The model under review builds one solid part; all positions refer to its coordinate system, in mm. Face numbers are marked on the shaded views. A direction names the side the tool comes from. Coordinates: 2 decimals unless noted, no trailing zeros. Loops run counter-clockwise (first coordinate to the right, second up) from the corner with the lowest first, then second, coordinate; pieces in that order, holes last. Notation, with made-up numbers: M 57.25,-20 L 82.25,-20 A28 ccw 82.25,11 Z; hole C 20.5,26 d6. An arc over 180 degrees is marked long. Use one line per item in the form item = value.
```python
from build123d import *

# Parameters (mm, degrees)
F1_DEPTH = 6.2484
F3_DEPTH = 0.9398
F4_W     = 24.0350353877
F4_H     = 1.27
F5_DEPTH = 1.27
F7_DEPTH = 9.145


with BuildPart() as f1:
    # F0 (on Top) → F1 (new body)
    with BuildSketch(Plane.XY):
        with BuildLine():
            Line((10.287, 4.572), (-23.3934, 4.572))
            Line((-23.3934, 4.572), (-23.3934, -4.572))
            Line((-23.3934, -4.572), (10.287, -4.572))
            ThreePointArc((10.287, -4.572), (14.859, 0), (10.287, 4.572))
        make_face()
    extrude(amount=F1_DEPTH)

    # F2 (on face) → F3 (cut)
    with BuildSketch(Plane(origin=(0, 4.572, 0), x_dir=(-1, 0, 0), z_dir=(0, 1, 0))):
        Polygon((23.3934, 6.2484), (-2.0066, 6.2484), (-0.6416353877, 4.064), (23.3934, 4.064), align=None)
    extrude(amount=-F3_DEPTH, mode=Mode.SUBTRACT)

    # F4 (on face) → F5 (cut)
    with BuildSketch(Plane(origin=(0, 3.6322, 0), x_dir=(-1, 0, 0), z_dir=(0, 1, 0))):
        with Locations((11.3758823062, 4.699)):
            Rectangle(F4_W, F4_H)
    extrude(amount=-F5_DEPTH, mode=Mode.SUBTRACT)

    # F6 (on face) → F7 (cut, through all)
    with BuildSketch(Plane(origin=(0, 4.572, 0), x_dir=(-1, 0, 0), z_dir=(0, 1, 0))):
        Polygon((19.4889663415, 6.2484), (23.3934, 0), (23.3934, 6.2484), align=None)
    extrude(amount=-F7_DEPTH, mode=Mode.SUBTRACT)

    # F8: F1 across plane


with BuildPart() as f1_1:
    add(f1.part)
    add(f1.part.mirror(Plane.XZ), mode=Mode.INTERSECT)

    # F9 (on Front) → F10 (revolve, cut)
    with BuildSketch(Plane.XZ):
        Polygon((3.4612531172, 5.5391628772), (0, 0), (-1.3459949312, -2.1540421642), (-0.3228249031, -2.7933897565), (4.4844231452, 4.8998152849), align=None)
        Polygon((5.7204784574, 9.154679198), (3.4612531172, 5.5391628772), (4.4844231452, 4.8998152849), (7.6917084592, 4.9278048398), (9.0377033903, 7.081847004), align=None)
    revolve(axis=Axis((2.8602392287, 0, 4.577339599), (0.5299192642, 0, 0.8480480962)), mode=Mode.SUBTRACT)


solid = f1_1.part
```
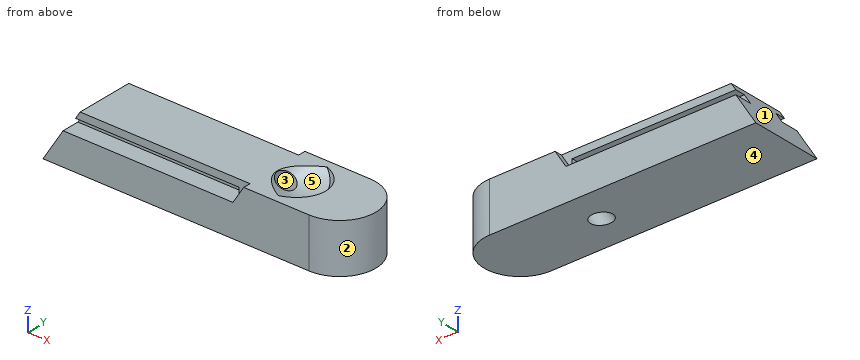
1. Add section C-C (x = 12.5). State the section outline as (y, z) points, then the cut area to 3 significant figures.
Response values:
outline = M -4,0 L 4,0 L 4,6.25 L -4,6.25 Z
area = 50.0 mm^2
2. Insertion check: P1, Ø1.4, axis at y = 3, z = 4.5, coming from the -X side; P2, Ø1.7, axis at x = -5, z = 5.5, coming from the -Y side; P3, Ø0.6, axis at x = -11, z = 4.5, coming from the -Y side. Each pin has a flat end and moves straight along its axis. Give the tip position at first contact, or say it passes through.
Response values:
P1 = -21.02
P2 = -3.63
P3 = -2.36
3. The part is to be moulded in two halves that separate along Y. For the marked faces 1, 2 and 3, say which applies: pulls with the +Y half, pulls with the -Y half, needs draft (parallel to the pull), parting line crosses it, or undercut.
Response values:
face_1 = needs draft
face_2 = parting line crosses it
face_3 = undercut
4. Add section A-A (y = 0). State the section outline as (x, z) points.
Response values:
outline = M -23.39,0 L -1.42,0 L 2.44,6.18 L 2.4,6.25 L -19.49,6.25 Z; M 1.42,0 L 14.86,0 L 14.86,6.25 L 8.52,6.25 L 7.69,4.93 L 4.48,4.9 Z
5. Wall thickness on line 1 along Z through (x, y) = (-0.5, 2.75); line 2 along X through (y, z) = (0.75, 4.5); line 3 along X through (y, z) = (0.25, 5.5): over which ranges is each line inside the solid? List them lowest first. Write a range as from..to.
Response values:
line_1 = 0..4.06, 5.33..6.25
line_2 = -20.58..1.7, 3.93..14.8
line_3 = -19.96..2.04, 8.04..14.85
6. Machinability: for the marked faces 4 and 5, which of the approach directions +Z, -Z, +X, -X, +Y, -Y give a long, thin tool a straight path to every point of the face, cutting with its end or side? Answer none if there is none.
Response values:
face_4 = -Z, +X, -X, +Y, -Y
face_5 = +Z
7. Add section B-B (x = -13). State the section outline as (y, z) points.
Response values:
outline = M -4.57,0 L 4.57,0 L 4.57,4.06 L 2.36,4.06 L 2.36,5.33 L 3.63,5.33 L 3.63,6.25 L -3.63,6.25 L -3.63,5.33 L -2.36,5.33 L -2.36,4.06 L -4.57,4.06 Z
